Answer from the drawing. Dimensions are ordinates in mm from the lowest x, y and z of the part. A direction names the side the tool comes from. Coordinates: 2 decimals unless noted, no trailing zeros. Write each loop counter-clockwise with the first axis right and the second up, starting at its lowest first coordinate (ties: lowest second). Pieces come first, ordered by that corner, then holes.
(1) Determine the mould class of the marked faces 3, 4, 5 and 6 for opening direction X: pulls with the +X half, pulls with the -X half, needs draft (parallel to the pull), parting line crosses it, or undercut.
(2) The part is cut by section C-C, the plane x = 5.25. Determine the outline of the cut face in (y, z), and give its area (3 significant figures).
(3) Given pin 1 (6.5 mm diameter, centred on x = 6.5, z = 11.5, fed in from +Y); pin 2 (3 mm diameter, centred on y = 4, z = 10.5, fed in from -X); pin 3 (2 mm diameter, centred on y = 3.5, z = 9, fed in from +X), each flat-ended and moving along its own axis, determine where each tip first touches the part or whether it passes through.
(4) Straight lines are drawn through the part: line 1 along X through (y, z) = (3.85, 14.5); line 2 along Y through (x, z) = (3.25, 15.75). For each, find the intervals that lie inside material, in ascending order.
(5) The part is cut by section B-B, the plane z = 7.25. Determine the outline of the cut face in (x, y).
(6) Which of the six approach directions +Z, -Z, +X, -X, +Y, -Y give full straight-line access (tool end or side, diameter ignored) to the marked faces 1 and 2?
(7) The part is cut by section A-A, the plane y = 4.2. Determine the outline of the cut face in (x, z).
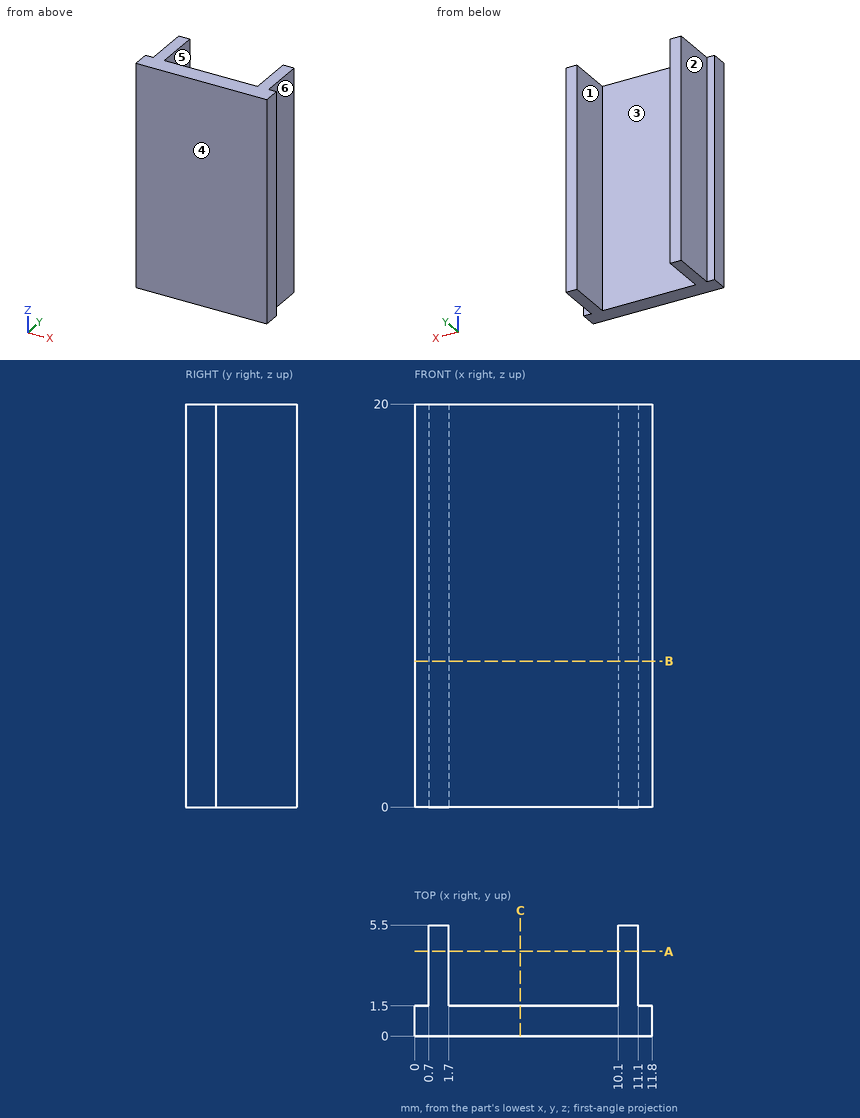
Computed:
1. face 3: undercut
1. face 4: needs draft
1. face 5: undercut
1. face 6: pulls with the +X half
2. outline: (0, 0) - (1.5, 0) - (1.5, 20) - (0, 20) - close
2. area: 30.0 mm2
3. pin 1: stops at y = 1.5
3. pin 2: stops at x = 0.7
3. pin 3: stops at x = 11.1
4. line 1: x = 0.7 to 1.7, 10.1 to 11.1
4. line 2: y = 0 to 1.5
5. outline: (0, 0) - (11.8, 0) - (11.8, 1.5) - (11.1, 1.5) - (11.1, 5.5) - (10.1, 5.5) - (10.1, 1.5) - (1.7, 1.5) - (1.7, 5.5) - (0.7, 5.5) - (0.7, 1.5) - (0, 1.5) - close
6. face 1: +Z, -Z, +Y
6. face 2: +Z, -Z, -X, +Y
7. outline: (0.7, 0) - (1.7, 0) - (1.7, 20) - (0.7, 20) - close; (10.1, 0) - (11.1, 0) - (11.1, 20) - (10.1, 20) - close
